For this review, take the finished solid that the model builds, in its own axes (mm). Coordinates: 2 decimals unless noted, no trailing zeros. Loops run counter-clockwise (first coordinate to the right, second up) from the corner with the lowest first, then second, coordinate; pieces in that order, holes last. Notation, with made-up numbers: (26, 57) - (78, 57) arc R33 cw to (78, 85) - close; hole circle Ø1 at (22, 15). An arc over 180 degrees is marked (long way). Answer as a JSON object with one key per item and string values. Group by question number.
Item 1: Mouldability with a two-part tool opening along Y and no side actions: class faces 1 (the flat face through (-2, -11.684, 1)), 2 (the flat face through (-14.395, 0, 1)), 3 (the cylindrical face through (-13.35, -1.88, 1.48)) as released by +Y, released by -Y, zero draft, split by the parting line, or undercut.
Item 2: We need section A-A (z = 1.8). Give the boundary of the cut face in (x, y).
Item 3: To check wall thickness, follow line 1 (Y direction, x = -12.25, z = 2.4); line 2 (Y direction, x = -13, z = 0.2). State the ranges of each line that lie inside material, in increasing order.
from build123d import *

# Parameters (mm, degrees)
SKETCH_1_W                = 25
SKETCH_1_H                = 24
EXTRUDE_1_DEPTH           = 3
HOLE_WIZARD_2_0_2_1_D     = 2
HOLE_WIZARD_2_0_2_1_DEPTH = 5.5
HOLE_WIZARD_2_0_2_1_TIP   = 0.600860619


with BuildPart() as part:
    # 草图1 → 凸台-拉伸1 (new body)
    with BuildSketch(Plane.XY):
        with Locations((-1.895437834, 0.316156105)):
            Rectangle(SKETCH_1_W, SKETCH_1_H)
    extrude(amount=EXTRUDE_1_DEPTH)

    # Ø2.0 (2) 直径孔1
    with Locations(Plane.XY.offset(3)):
        with Locations((-12.395437834, 10.316156105), (8.604562166, 10.316156105), (-12.395437834, -2.183843895), (8.604562166, -2.183843895)):
            Hole(HOLE_WIZARD_2_0_2_1_D / 2, depth=HOLE_WIZARD_2_0_2_1_DEPTH)
            with Locations((0, 0, -(HOLE_WIZARD_2_0_2_1_DEPTH + HOLE_WIZARD_2_0_2_1_TIP / 2))):  # 118° drill point
                Cone(0, HOLE_WIZARD_2_0_2_1_D / 2, HOLE_WIZARD_2_0_2_1_TIP, mode=Mode.SUBTRACT)


solid = part.part
Check sheet entries:
{
 "1": {"face 1": "released by -Y", "face 2": "zero draft", "face 3": "undercut"},
 "2": {"outline": "(-14.4, -11.68) - (10.6, -11.68) - (10.6, 12.32) - (-14.4, 12.32) - close; hole circle Ø2 at (-12.4, -2.18); hole circle Ø2 at (-12.4, 10.32); hole circle Ø2 at (8.6, -2.18); hole circle Ø2 at (8.6, 10.32)"},
 "3": {"line 1": "y = -11.68 to -3.17, -1.19 to 9.33, 11.31 to 12.32", "line 2": "y = -11.68 to -2.98, -1.39 to 9.52, 11.11 to 12.32"}
}
